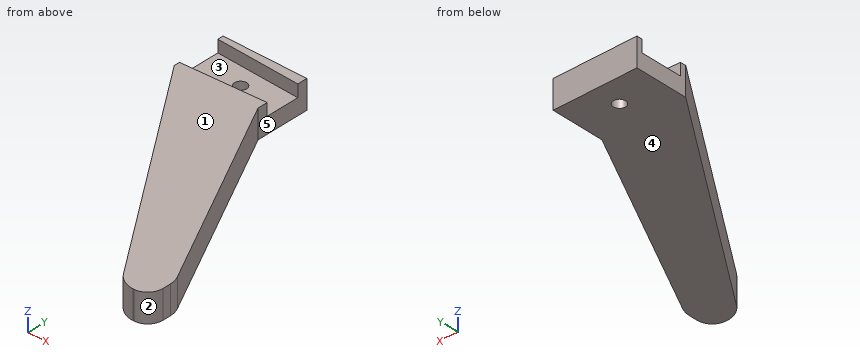
Autodesk Fusion 360 part; units mm, degrees
sketch "Sketch1" plane through (0, 0, 0) normal (0, 0, 1) x (1, 0, 0)
  line L0 (5.5, -3.5) -> (-5.5, -3.5)
  line L1 (-5.5, -3.5) -> (-5.5, 3.5)
  line L2 (-5.5, 3.5) -> (5.5, 3.5)
  line L3 (5.5, 3.5) -> (5.5, -3.5)
  line L4 (5.5, -3.5) -> (-5.5, 3.5) construction
  line L5 (-5.5, -3.5) -> (5.5, 3.5) construction
  line L6 (-5.5, 2.75) -> (-5.5, -2.75)
  line L7 (5.5, 2.2) -> (5.5, -2.2)
  line L8 (-5.5, 2.75) -> (5.5, 2.2)
  line L9 (-5.5, -2.75) -> (5.5, -2.2)
  circle A0 centre (0, 0) radius 0.8
  line L10 (-5.5, -3.5) -> (20, -3.5) construction
  line L11 (20, -31.9548) -> (20, -33)
  line L12 (18, -35) -> (17.9246, -35)
  line L13 (-5.5, -46.9761) -> (-5.5, -3.5) construction
  circle A1 centre (-12, 0) radius 47.4236 construction
  line L14 (0, 0) -> (-12, 0)
  line L15 (5.5, -3.5) -> (19.6582, -30.5642)
  line L16 (-5.5, -3.5) -> (15.4597, -33.7101)
  arc A2 (18, -35) -> (20, -33) centre (18, -33) ccw
  circle A3 centre (-12, 0) radius 46.596
  arc A4 (15.4597, -33.7101) -> (17.9246, -35) centre (17.9246, -32) ccw
  arc A5 (20, -31.9548) -> (19.6582, -30.5642) centre (17, -31.9548) ccw
  point P0 (-5.5, -35)
  dimension "d1" = 11
  dimension "d2" = 7
  dimension "d3" = 5.5
  dimension "d4" = 4.4
  dimension "d5" = 1.6
  dimension "d16" = 35
  dimension "d17" = 20
  dimension "d19" = 12
  dimension "d20" = 11.9761
  dimension "d21" = 2
  dimension "d22" = 3
extrude "Extrude1" add sketch "Sketch1" along normal blind 1.6 contours L0 L1 L3 L9 | L1 L2 L3 L8 makes body 1 at (-1.8333, 2.5667, 0.5333) makes body 2 at (-1.8333, -2.5667, 0.5333)
extrude "Extrude2" add sketch "Sketch1" against normal blind 2.1 contours L0 L1 L3 L9 | L1 L3 L6 L7 L8 L9 | L1 L2 L3 L8 bodies 2 1
extrude "Extrude5" add sketch "Sketch1" along normal up to surface (1.6 mm away) contours L0 L11 L12 L15 L16 A2 A3 A4 A5 bodies 2
extrude "Extrude6" add 1 faces at (5.1532, -13.57, 0) along direction (0, 0, -1) up to surface (2.1 mm away) on bodies 2 bodies 2
Here's how the part is built. I have some questions about the finished solid (model axes, mm). Face numbers are marked on the shaded views. A direction names the side the tool comes from. Round coordinates to 2 decimals unless told otherwise and drop trailing zeros. Order: outer loops, then holes, each group sorted by start corner. A loop starts at its lowest first (then second) coordinate and runs counter-clockwise, first axis right, second up. Notation, with made-up numbers: (23.25, 16.25) -> (72.25, 16.25) arc R8 ccw to (72.25, 30.25) -> close; hole circle Ø9 at (56.5, 31). An arc over 180 degrees is marked (long way). Return JSON: item names as keys, results as strings.
Q1. If we section it at A-A on z = -0.45: List the corners of the cut face in (x, y) for me, plus the area to 3 significant figures.
Filled sheet:
{"outline": "(-5.5, -3.5) -> (15.46, -33.71) arc R3 ccw to (17.92, -35) -> (18, -35) arc R2 ccw to (20, -33) -> (20, -31.95) arc R3 ccw to (19.66, -30.56) -> (5.5, -3.5) -> (5.5, 3.5) -> (-5.5, 3.5) -> close; hole circle Ø1.6 at (0, 0)", "area": "332 mm^2"}
Q2. For pin 1 Ø4.5 at (x, y) = (-0.5, 0) entering from +Z; pin 2 Ø1.5 at (y, z) = (-22, 1) entering from +X; pin 3 Ø2 at (y, z) = (-14.5, 0) entering from +X, each with a flat end and sliding along its axis, tell me the tip position at first contact or that it passes through.
Filled sheet:
{"pin 1": "stops at z = 0", "pin 2": "stops at x = 15.57", "pin 3": "stops at x = 11.78"}
Q3. If we section it at C-C on x = 0: List the corners of the cut face in (y, z) for me (3 decimals).
Filled sheet:
{"outline": "(-11.427, -2.1) -> (-0.8, -2.1) -> (-0.8, 0) -> (-2.475, 0) -> (-2.475, 1.6) -> (-11.427, 1.6) -> close; (0.8, -2.1) -> (3.5, -2.1) -> (3.5, 1.6) -> (2.475, 1.6) -> (2.475, 0) -> (0.8, 0) -> close"}
Q4. If we section it at B-B on y = 0: List the corners of the cut face in (x, z) for me.
Filled sheet:
{"outline": "(-5.5, -2.1) -> (-0.8, -2.1) -> (-0.8, 0) -> (-5.5, 0) -> close; (0.8, -2.1) -> (5.5, -2.1) -> (5.5, 0) -> (0.8, 0) -> close"}
Q5. Which directions (+Z, -Z, +X, -X, +Y, -Y) give clear straight access to the entire face, cutting with the end or side of a thin tool? Please do the marked faces 4 and 5.
Filled sheet:
{"face 4": "-Z, +X, -X, +Y, -Y", "face 5": "+Z, -Z, +X, +Y"}
Q6. If we mould it in two halves opening along Y, with no side actions, what happens to the marked faces 1, 2 and 3? For each: released by +Y, released by -Y, zero draft, split by the parting line, or undercut.
Filled sheet:
{"face 1": "zero draft", "face 2": "released by -Y", "face 3": "undercut"}
Q7. I need wall thicknesses on line 1 along X through (y, z) = (0, -0.75); line 2 along X through (y, z) = (-3, -0.6); line 3 along Y through (x, z) = (0.5, 0.15). Which ranges of each line are inside material? Lowest first, please. Write a range as from..to.
Filled sheet:
{"line 1": "x = -5.5..-0.8, 0.8..5.5", "line 2": "x = -5.5..5.5", "line 3": "y = -12.15..-2.45, 2.45..3.5"}
Q8. If we section it at D-D on x = -3.5: List the corners of the cut face in (y, z) for me, plus the area to 3 significant figures.
Filled sheet:
{"outline": "(-6.38, -2.1) -> (3.5, -2.1) -> (3.5, 1.6) -> (2.65, 1.6) -> (2.65, 0) -> (-2.65, 0) -> (-2.65, 1.6) -> (-6.38, 1.6) -> close", "area": "28.1 mm^2"}
